For this review, take the finished solid that the model builds, in its own axes (mm). Coordinates: 2 decimals unless noted, no trailing zeros. Loops run counter-clockwise (first coordinate to the right, second up) from the corner with the lowest first, then second, coordinate; pieces in that order, holes last. Notation, with made-up numbers: M 23.5,64 L 35.5,64 A18 cw 35.5,91 Z; hole C 82.5,81.5 d8. An arc over 180 degrees is marked long. Use one line per item in the form item = value.
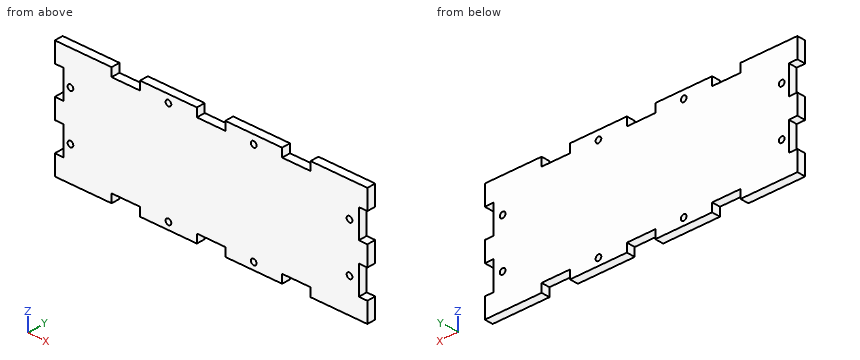
```python
from build123d import *

# Parameters (mm, degrees)
F0_R     = 1
F1_DEPTH = 3


with BuildPart() as f1:
    # F0 (on Front) → F1 (new body)
    with BuildSketch(Plane.XZ):
        Polygon((-51.973995, 1.919852), (-54.973995, 1.919852), (-54.973995, -1.580148), (-54.973995, -5.080148), (-51.973995, -5.080148), (-51.973995, -15.080148), (-54.973995, -15.080148), (-54.973995, -22.080148), (-34.973995, -22.080148), (-34.973995, -19.080148), (-24.973995, -19.080148), (-24.973995, -22.080148), (-4.973995, -22.080148), (-4.973995, -19.080148), (0.026005, -19.080148), (5.026005, -19.080148), (5.026005, -22.080148), (25.026005, -22.080148), (25.026005, -19.080148), (35.026005, -19.080148), (35.026005, -22.080148), (55.026005, -22.080148), (55.026005, -15.080148), (52.026005, -15.080148), (52.026005, -5.080148), (55.026005, -5.080148), (55.026005, -1.580148), (55.026005, 1.919852), (52.026005, 1.919852), (52.026005, 11.919852), (55.026005, 11.919852), (55.026005, 18.919852), (35.026005, 18.919852), (35.026005, 15.919852), (25.026005, 15.919852), (25.026005, 18.919852), (5.026005, 18.919852), (5.026005, 15.919852), (0.026005, 15.919852), (-4.973995, 15.919852), (-4.973995, 18.919852), (-24.973995, 18.919852), (-24.973995, 15.919852), (-34.973995, 15.919852), (-34.973995, 18.919852), (-54.973995, 18.919852), (-54.973995, 11.919852), (-51.973995, 11.919852), align=None)
        with Locations((-14.973995, -19.580148)):
            Circle(F0_R, mode=Mode.SUBTRACT)
        with Locations((-49.451287, -10.080148)):
            Circle(F0_R, mode=Mode.SUBTRACT)
        with Locations((15.026005, -19.580148)):
            Circle(F0_R, mode=Mode.SUBTRACT)
        with Locations((48.736135, -10.080148)):
            Circle(F0_R, mode=Mode.SUBTRACT)
        with Locations((-49.451287, 6.919852)):
            Circle(F0_R, mode=Mode.SUBTRACT)
        with Locations((-14.973995, 16.168253)):
            Circle(F0_R, mode=Mode.SUBTRACT)
        with Locations((48.736135, 6.919852)):
            Circle(F0_R, mode=Mode.SUBTRACT)
        with Locations((15.026005, 15.900204)):
            Circle(F0_R, mode=Mode.SUBTRACT)
    extrude(amount=F1_DEPTH)


solid = f1.part
```
1. Consider section B-B on x = -30. Write out the cut boundary in (y, z).
Computed values:
outline = M -3,-19.08 L 0,-19.08 L 0,15.92 L -3,15.92 Z
2. Wall thickness on line 1 along X through (y, z) = (-1.45, 16); line 2 along X through (y, z) = (-0.3, 7); line 3 along Z through (x, y) = (15, -2.6): over which ranges is each line inside the solid? List them lowest first. Write a range as from..to.
Computed values:
line_1 = -54.97..-34.97, -24.97..-15.96, -13.99..-4.97, 5.03..14.03, 16.02..25.03, 35.03..55.03
line_2 = -51.97..-50.45, -48.45..47.74, 49.73..52.03
line_3 = -22.08..-20.58, -18.58..14.9, 16.9..18.92
3. Consider section C-C on y = -0.8. State how many separate pieces and enclosed holes the cut face has, plus the area to 3 significant figures.
Computed values:
separate_pieces = 1
enclosed_holes = 8
area = 4,180 mm2
4. Consider section A-A on z = 3.5. Write out the cut boundary in (x, y), plus the area to 3 significant figures.
Computed values:
outline = M -51.97,-3 L 52.03,-3 L 52.03,0 L -51.97,0 Z
area = 312 mm2
5. For pin 1 Ø1.5 at (x, y) = (-29, -1.5) entering from +Z; pin 2 Ø1.6 at (x, z) = (-14.97, -19.58) entering from +Y; pin 3 Ø0.9 at (x, y) = (31.5, -1.5) entering from -Z; pin 4 Ø1.5 at (y, z) = (-2, 9.5) entering from -X, all flat-tipped, find the tip position at first contact; note any pin that passes through.
Computed values:
pin_1 = 15.92
pin_2 = through
pin_3 = -19.08
pin_4 = -51.97
